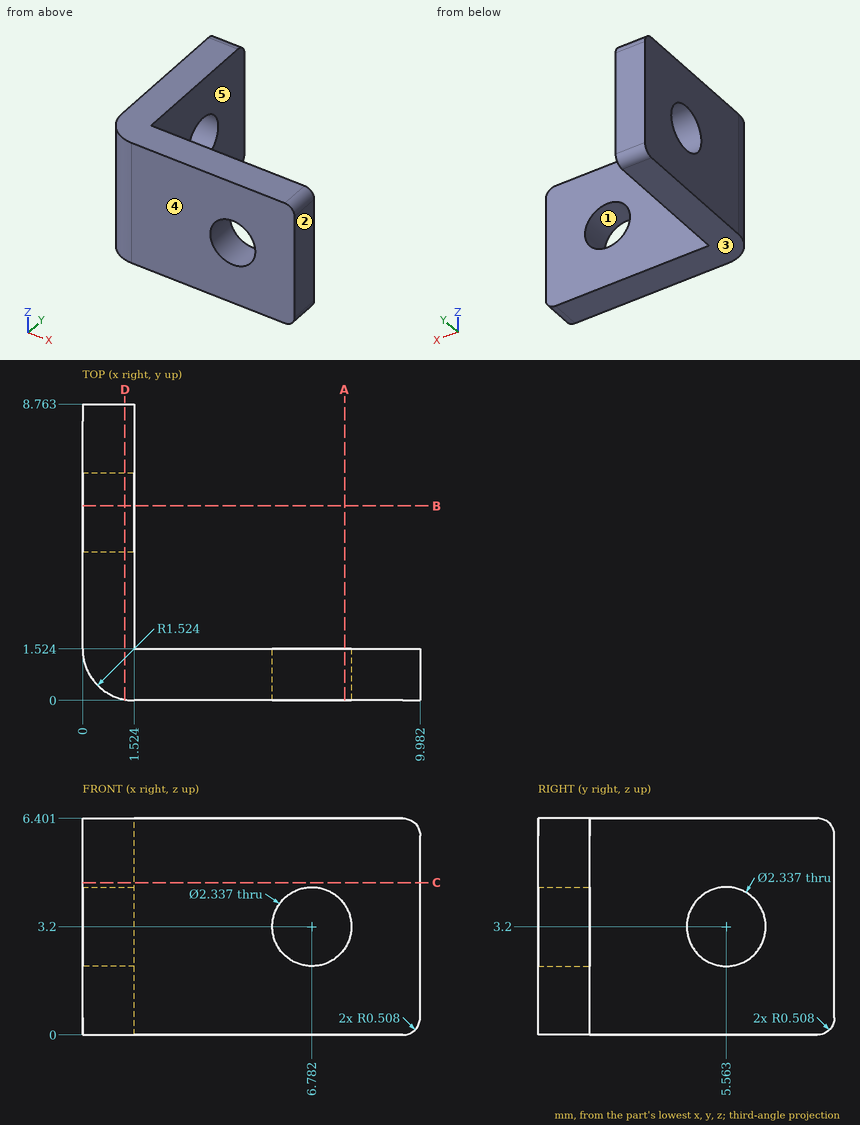
For this review, use the dimensioned drawing (mm, ordinates from the lowest corner) and the shaded views. A direction names the side the tool comes from. Give positions to 0.01 mm unless a question says otherwise; leave off trailing zeros. Order: outer loops, then holes, each group sorted by start corner. A loop starts at its lowest first (then second) coordinate and runs counter-clockwise, first axis right, second up. Notation, with made-up numbers: (10, -38.5) - (59, -38.5) arc R20 cw to (59, -15.5) - close; hole circle Ø9 at (-8.5, -17). An arc over 180 degrees is marked (long way). Use a Markdown table: item, result. Add a question column.
(1) Wall thickness on probe 1 along X at (y, z) = (1, 4.25) (1 decimal); probe 2 along Y at (x, z) = (3.75, 1.5): over which ranges is each line inside the solid? List them lowest first. Write a range as [from, to].
(2) Add section C-C on z = 4.5. Give the boundary of the cut face in (x, y).
(3) Add section A-A on x = 7.75. Give the boundary of the cut face in (y, z) (1 decimal).
(4) Add section B-B on y = 5.75. Give the boundary of the cut face in (x, z).
(5) Add section D-D on x = 1.25. Give the boundary of the cut face in (y, z) (1 decimal).
(6) Clearance check with flat-ended pins moving along their axes: P1, Ø1.9, axis at y = 6, z = 2.5, coming from the +X side; P2, Ø3.5, axis at x = 6.78, z = 3.2, coming from the +Y side. State where each tip first meets the part, or that it passes through.
(7) Machinability: for the marked faces 4 and 5, which of the approach directions +Z, -Z, +X, -X, +Y, -Y give a long, thin tool a straight path to every point of the face, cutting with its end or side? Answer none if there is none.
(8) Mouldability with a two-part tool opening along Z and no side actions: class the marked faces 1, 2 and 3 as +Z half, -Z half, draft (parallel to the pull), parting line (faces both ways), or undercut.
Report:
| question | item | result |
|---|---|---|
| 1 | probe 1 | x = [0.1, 6.3], [7.3, 10] |
| 1 | probe 2 | y = [0, 1.52] |
| 2 | outline | (0, 1.52) arc R1.52 ccw to (1.52, 0) - (9.98, 0) - (9.98, 1.52) - (1.52, 1.52) - (1.52, 8.76) - (0, 8.76) - close |
| 3 | outline | (0, 0) - (1.5, 0) - (1.5, 2.5) - (0, 2.5) - close; (0, 3.9) - (1.5, 3.9) - (1.5, 6.4) - (0, 6.4) - close |
| 4 | outline | (0, 0) - (1.52, 0) - (1.52, 2.05) - (0, 2.05) - close; (0, 4.35) - (1.52, 4.35) - (1.52, 6.4) - (0, 6.4) - close |
| 5 | outline | (0, 0) - (8.3, 0) arc R0.5 ccw to (8.8, 0.5) - (8.8, 5.9) arc R0.5 ccw to (8.3, 6.4) - (0, 6.4) - close; hole circle Ø2.3 at (5.6, 3.2) |
| 6 | P1 | stops at x = 1.52 |
| 6 | P2 | stops at y = 1.52 |
| 7 | face 4 | +Z, -Z, +X, -X, -Y |
| 7 | face 5 | +Z, -Z, +X, +Y |
| 8 | face 1 | undercut |
| 8 | face 2 | draft |
| 8 | face 3 | -Z half |
